For this review, use the dimensioned drawing (mm, ordinates from the lowest corner) and the shaded views. A direction names the side the tool comes from. Give positions to 0.01 mm unless a question says otherwise; leave off trailing zeros. Order: outer loops, then holes, each group sorted by start corner. A loop starts at its lowest first (then second) coordinate and runs counter-clockwise, first axis right, second up. Notation, with made-up numbers: M 40.25,7 L 94.25,7 A8 cw 94.25,13 Z; hole C -36,57.25 d1. An arc over 180 degrees is marked long. Answer as CSV lines item,"result". Start each with the question number.
1. Clearance check with flat-ended pins moving along their axes: P1, Ø1.3, axis at x = 5.5, y = 1, coming from the +Z side (1 decimal); P2, Ø1.7, axis at x = 4.5, y = 18.5, coming from the -Z side; P3, Ø2, axis at x = 2, z = 10.5, coming from the -Y side; P4, Ø8, axis at y = 14.5, z = 36.5, coming from the +X side. State where each tip first meets the part, or that it passes through.
2. We need section B-B, the plane y = 12.25. Give the boundary of the cut face in (x, z) (1 decimal).
3. We need section C-C, the plane z = 57.5. Give the boundary of the cut face in (x, y) (1 decimal), and give its area (3 significant figures).
4. Machinability: for the marked faces 1, 2, 3, 4 and 5, which of the approach directions +Z, -Z, +X, -X, +Y, -Y give a long, thin tool a straight path to every point of the face, cutting with its end or side? Answer none if there is none.
5. For line 1 along Y through (x, z) = (1.5, 63.5); line 2 along Z through (x, y) = (5.5, 16.25) (1 decimal); line 3 along Y through (x, z) = (4.25, 11.5), list the stretches that pass through material, from the lowest coordinate up.
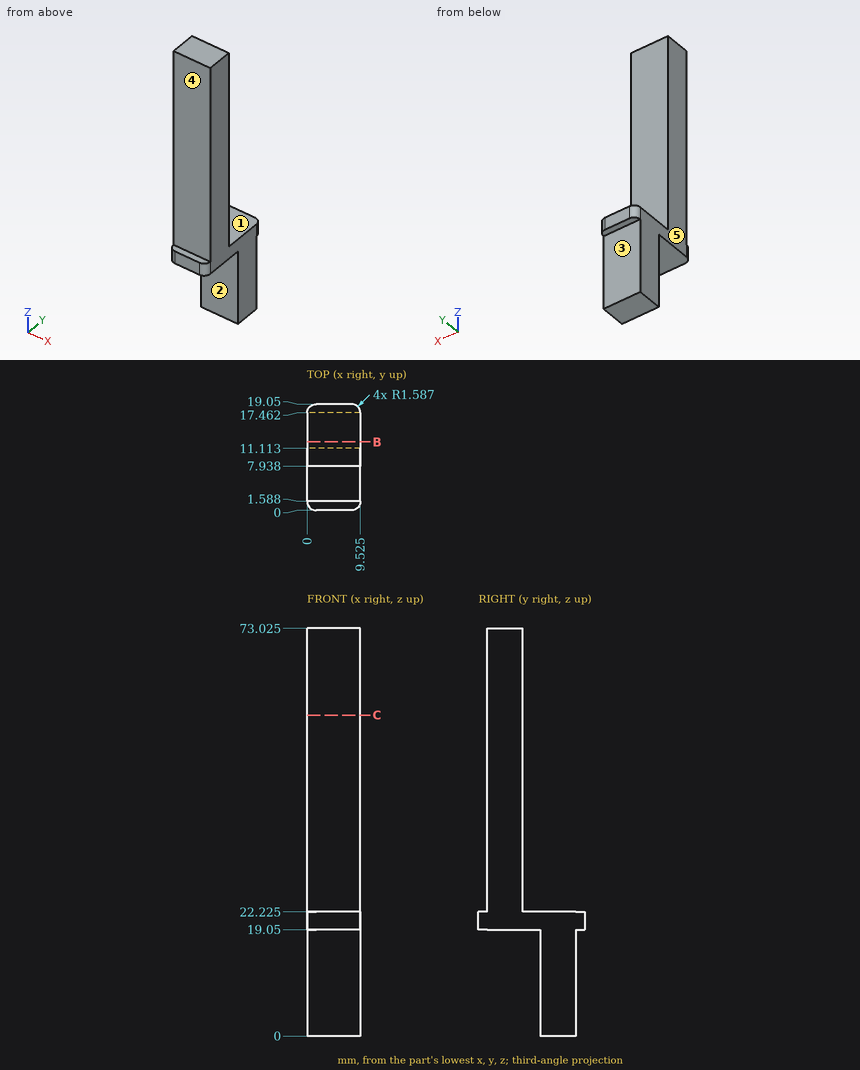
Result set:
1,P1,"z = 73"
1,P2,"z = 19.05"
1,P3,"y = 11.11"
1,P4,"through"
2,outline,"M 0,0 L 9.5,0 L 9.5,22.2 L 0,22.2 Z"
3,outline,"M 0,1.6 L 9.5,1.6 L 9.5,7.9 L 0,7.9 Z"
3,area,"60.5 mm2"
4,face 1,"+Z, +X, -X, +Y"
4,face 2,"-Z, +X, -X, -Y"
4,face 3,"-Z, +X, -X, +Y"
4,face 4,"+Z, +X, -X, -Y"
4,face 5,"+Z, -Z, -X, +Y, -Y"
5,line 1,"1.59 to 7.94"
5,line 2,"0 to 22.2"
5,line 3,"11.11 to 17.46"
